from build123d import *

# Parameters (mm, degrees)
BOSS_EXTRU_1_DEPTH      = 15
ESQUISSE2_R             = 1.55
ESQUISSE2_W             = 15
ESQUISSE2_H             = 10
BOSS_EXTRU_2_DEPTH      = 4
ESQUISSE5_R             = 2.05
ENL_V_MAT_EXTRU_3_DEPTH = 129.379320765
ESQUISSE7_W             = 114
ESQUISSE7_H             = 5
BOSS_EXTRU_3_DEPTH      = 5
CONG_1_R                = 1.5
CONG_1_OF_SYM_TRIE5_R   = 1.5


with BuildPart() as part:
    # Esquisse1 → Boss.-Extru.1 (new body)
    with BuildSketch(Plane.XY):
        Polygon((0, 10), (0, 5), (0, 0), (114, 0), (114, 10), align=None)
    boss_extru_1 = extrude(amount=BOSS_EXTRU_1_DEPTH)

    # Esquisse2 → Boss.-Extru.2 (add)
    # profile 1 of 2: a face of its own
    with BuildSketch(Plane(origin=(114, 0, 0), x_dir=(0, 0, -1), z_dir=(1, 0, 0))):
        with BuildLine():
            ThreePointArc((0, 29), (-4.629874257, 35.929096494), (-12.803300859, 34.303300859))
            Line((-12.803300859, 34.303300859), (-32.803300859, 14.303300859))
            ThreePointArc((-32.803300859, 14.303300859), (-34.429096494, 11.870125743), (-35, 9))
            Line((-35, 9), (-35, 0))
            Line((-35, 0), (-15, 0))
            Line((-15, 0), (-15, 10))
            Line((-15, 10), (0, 10))
            Line((0, 10), (0, 29))
        make_face()
        with Locations((-27.5, 9)):
            Circle(ESQUISSE2_R, mode=Mode.SUBTRACT)
        with Locations((-7.5, 29)):
            Circle(ESQUISSE2_R, mode=Mode.SUBTRACT)
    # profile 2 of 2: a face of its own
    with BuildSketch(Plane(origin=(114, 0, 0), x_dir=(0, 0, -1), z_dir=(1, 0, 0))):
        with Locations((-7.5, 5)):
            Rectangle(ESQUISSE2_W, ESQUISSE2_H)
    boss_extru_2 = extrude(amount=BOSS_EXTRU_2_DEPTH)

    # Esquisse5 → Enlèv. mat.-Extru.3 (cut, through all)
    with BuildSketch(Plane.XZ):
        with Locations(Location((8, 5, 0), (0, 0, 270))):
            Circle(ESQUISSE5_R)
        with Locations(Location((72, 5, 0), (0, 0, 270))):
            Circle(ESQUISSE5_R)
        with Locations((88, 5)):
            Circle(ESQUISSE5_R)
    enl_v_mat_extru_3 = extrude(amount=-ENL_V_MAT_EXTRU_3_DEPTH, mode=Mode.SUBTRACT)

    # Esquisse7 → Boss.-Extru.3 (add)
    with BuildSketch(Plane(origin=(0, 10, 0), x_dir=(1, 0, 0), z_dir=(0, 1, 0))):
        with Locations((57, -12.5)):
            Rectangle(ESQUISSE7_W, ESQUISSE7_H)
    boss_extru_3 = extrude(amount=BOSS_EXTRU_3_DEPTH)

    # Congé1
    cong_1_edges = [part.edges().sort_by_distance(p)[0] for p in [
        (114, 35.929096494, 4.629874257),
        (114, 24.303300859, 22.803300859),
        (114, 11.870125743, 34.429096494),
        (114, 4.5, 35),
        (118, 14.5, 0),
        (114, 19.5, 0),
        (118, 35.929096494, 4.629874257),
        (118, 24.303300859, 22.803300859),
        (118, 11.870125743, 34.429096494),
        (118, 4.5, 35),
        (57, 0, 15),
        (57, 15, 10),
        (57, 15, 15),
        (57, 10, 10),
        (57, 10, 0),
    ]]
    fillet(cong_1_edges, radius=CONG_1_R)

    # Symétrie5: Boss.-Extru.1, Boss.-Extru.2, Enlèv. mat.-Extru.3, Boss.-Extru.3 across plane
    add(boss_extru_1.mirror(Plane(origin=(0, 5, 15), x_dir=(0, 0, 1), z_dir=(1, 0, 0))))
    add(boss_extru_2.mirror(Plane(origin=(0, 5, 15), x_dir=(0, 0, 1), z_dir=(1, 0, 0))))
    add(enl_v_mat_extru_3.mirror(Plane(origin=(0, 5, 15), x_dir=(0, 0, 1), z_dir=(1, 0, 0))), mode=Mode.SUBTRACT)
    add(boss_extru_3.mirror(Plane(origin=(0, 5, 15), x_dir=(0, 0, 1), z_dir=(1, 0, 0))))

    # Congé1 of Symétrie5
    cong_1_of_sym_trie5_edges = [part.edges().sort_by_distance(p)[0] for p in [
        (-114, 35.929096494, 4.629874257),
        (-114, 24.303300859, 22.803300859),
        (-114, 11.870125743, 34.429096494),
        (-114, 4.5, 35),
        (-118, 14.5, 0),
        (-114, 19.5, 0),
        (-118, 35.929096494, 4.629874257),
        (-118, 24.303300859, 22.803300859),
        (-118, 11.870125743, 34.429096494),
        (-118, 4.5, 35),
        (-57, 0, 15),
        (-57, 15, 10),
        (-57, 15, 15),
        (-57, 10, 10),
        (-57, 10, 0),
    ]]
    fillet(cong_1_of_sym_trie5_edges, radius=CONG_1_OF_SYM_TRIE5_R)


solid = part.part
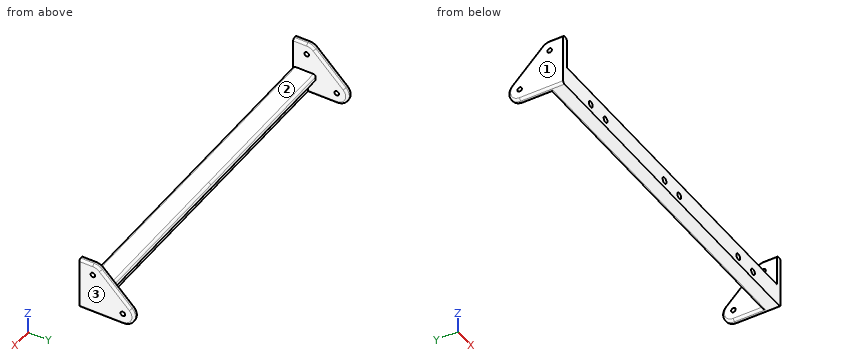
Read the model definition and answer for the solid it produces. Units are mm, in the model's axes. Face numbers are marked on the shaded views. Coordinates: 2 decimals unless noted, no trailing zeros. Loops run counter-clockwise (first coordinate to the right, second up) from the corner with the lowest first, then second, coordinate; pieces in that order, holes last. Notation, with made-up numbers: (47, 26) -> (78, 26) arc R17 ccw to (78, 43) -> close; hole circle Ø5 at (88.5, 48). An arc over 180 degrees is marked (long way). Write item = value, one per line. Start each with the question number.
1) Find the intervals of material crossed by L1, parallel to Z at x = -72, y = 4.75; L2, parallel to X at y = 17.5, z = 13, in increasing order. Write a range as from..to.
2) The mould has two halves that part along X. Classify the marked faces 1, 2 and 3: pulls with the +X half, pulls with the -X half, needs draft (parallel to the pull), parting line crosses it, or undercut.
3) The part is cut by section B-B, the plane x = -49. Determine the outline of the cut face in (y, z).
4) The part is cut by section A-A, the plane x = -8. Determine the outline of the cut face in (y, z).
5) Given P1, Ø3.5, axis at x = -52.5, z = 4.5, coming from the +Y side; P2, Ø0.6, axis at x = 33.5, z = 12.5, coming from the +Y side; P3, Ø12, axis at x = 75.5, z = 20, coming from the +Y side, each flat-ended and moving along its own axis, determine where each tip first touches the part or whether it passes through.
Result:
q1.L1 = 0..2.95, 7.05..15
q1.L2 = -118..-114, 114..118
q2.face_1 = pulls with the -X half
q2.face_2 = undercut
q2.face_3 = pulls with the +X half
q3.outline = (0, 0) -> (8.5, 0) arc R1.5 ccw to (10, 1.5) -> (10, 8.5) arc R1.5 cw to (11.5, 10) -> (13.5, 10) arc R1.5 ccw to (15, 11.5) -> (15, 13.5) arc R1.5 ccw to (13.5, 15) -> (1.5, 15) arc R1.5 ccw to (0, 13.5) -> close
q4.outline = (0, 0) -> (8.5, 0) arc R1.5 ccw to (10, 1.5) -> (10, 2.95) -> (0, 2.95) -> close; (0, 7.05) -> (10, 7.05) -> (10, 8.5) arc R1.5 cw to (11.5, 10) -> (13.5, 10) arc R1.5 ccw to (15, 11.5) -> (15, 13.5) arc R1.5 ccw to (13.5, 15) -> (1.5, 15) arc R1.5 ccw to (0, 13.5) -> close
q5.P1 = 10
q5.P2 = 15
q5.P3 = 14.91
